Geometry: final body of the model. Coordinates: model frame, mm. A direction names the side the tool comes from. Give positions to 0.01 mm unless a question says otherwise; leave off trailing zeros. Loops run counter-clockwise (first coordinate to the right, second up) from the corner with the lowest first, then second, coordinate; pieces in that order, holes last.
1. Section C-C, the plane y = 6. Output: boundary loops of the cut face in (x, z).
2. Draft query along Z for faces 1 (the face through (0, -9, 0)), 2 (the face through (0, 60.512, -55)), 3 (the face through (25, 2, -56)), 4 (the face through (2, -5, -120)). Return one class per face: +Z half, -Z half, draft (parallel to the pull), parting line (faces both ways), or undercut.
3. Material intervals for line 1 along Y through (x, z) = (0, -116.25); line 2 along Z through (x, y) = (-14, -11.5); line 3 along X through (y, z) = (15, -104), sorted ascending.
4. Access query for faces 5 (the face through (6.007, 50.372, -35.924)), 6 (the face through (2, -5, 10)), 7 (the face through (0, -9, -110)). Directions: +Z, -Z, +X, -X, +Y, -Y. A direction counts if a zero-diameter tool reaches every point of the face in a straight line with its end or side. Return the directions, or none.
5. First-contact query: P1, Ø11.5, axis at x = 0, y = -30, coming from the +Z side; P2, Ø1, axis at y = 1.5, z = -43, coming from the -X side; P3, Ø11, axis at x = 28.5, z = -85, coming from the -Y side; P4, Ø1, axis at x = -20.5, z = -74, coming from the -Y side. Flat tips, straight axial feed; report the tip coordinate or a pass-through.
6. Section D-D, the plane z = -55. Output: boundary loops of the cut face in (x, y), then the cut area to 3 significant figures.
7. Section A-A, the plane x = 0. Output: boundary loops of the cut face in (y, z).
8. Section B-B, the plane y = -30. Output: boundary loops of the cut face in (x, z).
from build123d import *

# Parameters (mm, degrees)
SKETCH1_R           = 5
BOSS_EXTRUDE1_DEPTH = 10
BOSS_EXTRUDE2_DEPTH = 55
SKETCH3_R           = 20
BOSS_EXTRUDE3_DEPTH = 20
SKETCH4_W           = 130
SKETCH4_H           = 65.511911844
BOSS_EXTRUDE4_DEPTH = 5


with BuildPart() as part:
    # Sketch1 → Boss-Extrude1 (new body)
    with BuildSketch(Plane.XY):
        with BuildLine():
            Line((-30, 40.511911844), (30, 40.511911844))
            Line((30, 40.511911844), (30, -25))
            ThreePointArc((30, -25), (22.67766953, -42.67766953), (5, -50))
            Line((5, -50), (-5, -50))
            ThreePointArc((-5, -50), (-22.67766953, -42.67766953), (-30, -25))
            Line((-30, -25), (-30, 40.511911844))
        make_face()
        with Locations((0, -30)):
            Circle(SKETCH1_R, mode=Mode.SUBTRACT)
    boss_extrude1 = extrude(amount=BOSS_EXTRUDE1_DEPTH)

    # Sketch2 → Boss-Extrude2 (add)
    with BuildSketch(Plane(origin=(0, 0, 0), x_dir=(-1, 0, 0), z_dir=(0, 0, -1))):
        Polygon((-30, 40.511911844), (-30, -25), (-25, -25), (-25, 30.511911844), (30, 30.511911844), (30, 40.511911844), align=None)
    boss_extrude2 = extrude(amount=BOSS_EXTRUDE2_DEPTH)

    # Mirror1: Boss-Extrude1, Boss-Extrude2 across plane
    add(boss_extrude1.mirror(Plane(origin=(0, 0, -55), x_dir=(1, 0, 0), z_dir=(0, 0, -1))))
    add(boss_extrude2.mirror(Plane(origin=(0, 0, -55), x_dir=(1, 0, 0), z_dir=(0, 0, -1))))

    # Sketch3 → Boss-Extrude3 (add)
    with BuildSketch(Plane(origin=(0, 40.511911844, 0), x_dir=(1, 0, 0), z_dir=(0, 1, 0))):
        with Locations(Location((0, 55, 0), (0, 0, 270))):
            Circle(SKETCH3_R)
    extrude(amount=BOSS_EXTRUDE3_DEPTH)

    # Sketch4 → Boss-Extrude4 (add)
    with BuildSketch(Plane(origin=(30, 0, 0), x_dir=(0, 0, -1), z_dir=(1, 0, 0))):
        with Locations((55, 7.755955922)):
            Rectangle(SKETCH4_W, SKETCH4_H)
    extrude(amount=BOSS_EXTRUDE4_DEPTH)


solid = part.part
Answers below:
1. outline: (-30, -120) - (35, -120) - (35, 10) - (-30, 10) - (-30, 0) - (25, 0) - (25, -110) - (-30, -110) - close
2. face 1: undercut
2. face 2: draft
2. face 3: undercut
2. face 4: -Z half
3. line 1: y = -50 to -35, -25 to 40.51
3. line 2: z = -120 to -110, 0 to 10
3. line 3: x = 25 to 35
4. face 5: +Y
4. face 6: +Z, +X, -X, +Y, -Y
4. face 7: -X, -Y
5. P1: stops at z = 10
5. P2: stops at x = 25
5. P3: stops at y = -25
5. P4: stops at y = 30.51
6. outline: (-30, 30.51) - (25, 30.51) - (25, -25) - (35, -25) - (35, 40.51) - (20, 40.51) - (20, 60.51) - (-20, 60.51) - (-20, 40.51) - (-30, 40.51) - close
6. area: 2,010 mm2
7. outline: (-50, -120) - (-35, -120) - (-35, -110) - (-50, -110) - close; (-50, 0) - (-35, 0) - (-35, 10) - (-50, 10) - close; (-25, -120) - (40.51, -120) - (40.51, -75) - (60.51, -75) - (60.51, -35) - (40.51, -35) - (40.51, 10) - (-25, 10) - (-25, 0) - (30.51, 0) - (30.51, -110) - (-25, -110) - close
8. outline: (-29.49, -120) - (-5, -120) - (-5, -110) - (-29.49, -110) - close; (-29.49, 0) - (-5, 0) - (-5, 10) - (-29.49, 10) - close; (5, -120) - (29.49, -120) - (29.49, -110) - (5, -110) - close; (5, 0) - (29.49, 0) - (29.49, 10) - (5, 10) - close
